Design review of the part built by this model. Coordinates are the model's own, in mm. Coordinates: 2 decimals unless noted, no trailing zeros. Loops run counter-clockwise (first coordinate to the right, second up) from the corner with the lowest first, then second, coordinate; pieces in that order, holes last. Notation, with made-up numbers: (48.25, -31) -> (106.25, -31) arc R10 cw to (106.25, -18) -> close; hole circle Ø1 at (37.25, -15.75). An arc over 180 degrees is marked (long way). Use a Markdown table: item, result. Add a question column.
Q1. Take a section at A-A on z = 2. Write out the cut boundary in (x, y), plus the area to 3 significant figures.
Q2. Take a section at B-B on y = -5. Write out the cut boundary in (x, z), plus the area to 3 significant figures.
Q3. Take a section at D-D on y = -3.5. Write out the cut boundary in (x, z).
Q4. For probe 1 along Z at (x, y) = (5, -5.1); probe 2 along X at (y, z) = (-5.55, 2); probe 3 along Z at (x, y) = (5.5, -4.25), list the stretches that pass through material, from the lowest coordinate up.
Q5. Clearance check with flat-ended pins moving along their axes: pin 1 Ø1.2 at (x, z) = (5, 2.5) entering from +Y; pin 2 Ø1.2 at (x, z) = (4.5, 2) entering from -Y. State where each tip first meets the part, or that it passes through.
Q6. Draft analysis for pull direction Z (two halves, no side actions). For faces 1 (the face through (5, -6, 3)), 2 (the face through (5, -6, 0)), 3 (the face through (4.93, -0.887, 0.761)), state which applies: pulls with the +Z half, pulls with the -Z half, needs draft (parallel to the pull), parting line crosses it, or undercut.
Q7. Take a section at C-C on x = 3.5. Write out the cut boundary in (y, z).
Solid Edge part; units mm, degrees
sketch "Sketch1" plane through (0, 0, 0) normal (-1, 0, 0) x (0, -1, 0)
  line L0 (10.25, 1.5) -> (2.1916, 1.5)
  line L1 (2.1916, 1.5) -> (1.75, 1.5)
  line L2 (1.75, 1.5) -> (0, 0)
  line L3 (0, 0) -> (12, 0)
  line L4 (10.25, 1.5) -> (12, 0)
extrude "Protrusion1" add sketch "Sketch1" against normal blind 10
sketch "Sketch2" plane through (0, 0, 0) normal (0, 1, 0) x (-1, 0, 0)
  line L0 (-8.25, 1.5) -> (-10, 0)
  line L1 (-10, 0) -> (-10, 1.5)
  line L2 (-10, 1.5) -> (-8.25, 1.5)
  line L3 (-1.75, 1.5) -> (0, 0)
  line L4 (0, 1.5) -> (0, 0)
  line L5 (-1.75, 1.5) -> (0, 1.5)
extrude "Recorte_Extrudado_1" cut sketch "Sketch2" against normal blind 12.6
sketch "Sketch3" plane through (0, -4.5, 0) normal (0, 1, 0) x (-1, 0, 0)
  circle A0 centre (-5, 2) radius 1
extrude "Protrusion2" add sketch "Sketch3" against normal blind 3
sketch "Sketch4" plane through (5, -4.5, 2.25) normal (0, 1, 0) x (-1, 0, 0)
  circle A0 centre (0, -0.25) radius 0.5
extrude "Cutout1" cut sketch "Sketch4" against normal blind 3
Answer list:
| question | item | result |
|---|---|---|
| 1 | outline | (4, -7.5) -> (4.5, -7.5) -> (4.5, -4.5) -> (4, -4.5) -> close; (5.5, -7.5) -> (6, -7.5) -> (6, -4.5) -> (5.5, -4.5) -> close |
| 1 | area | 3.00 mm² |
| 2 | outline | (0, 0) -> (10, 0) -> (8.25, 1.5) -> (5.87, 1.5) arc R1 ccw (long way) to (4.13, 1.5) -> (1.75, 1.5) -> close; hole circle Ø1 at (5, 2) |
| 2 | area | 14.1 mm² |
| 3 | outline | (0, 0) -> (10, 0) -> (8.25, 1.5) -> (1.75, 1.5) -> close |
| 4 | probe 1 | 0 to 1.5, 2.5 to 3 |
| 4 | probe 2 | 4 to 4.5, 5.5 to 6 |
| 4 | probe 3 | 0 to 1.5 |
| 5 | pin 1 | y = -4.5 |
| 5 | pin 2 | y = -10.37 |
| 6 | face 1 | undercut |
| 6 | face 2 | pulls with the -Z half |
| 6 | face 3 | pulls with the +Z half |
| 7 | outline | (-12, 0) -> (0, 0) -> (-1.75, 1.5) -> (-10.25, 1.5) -> close |
